Geometry check sheet. Reference: the model listing, model coordinates, mm. Face numbers are marked on the shaded views. A direction names the side the tool comes from. Give positions to 0.01 mm unless a question says otherwise; leave off trailing zeros. Loops run counter-clockwise (first coordinate to the right, second up) from the corner with the lowest first, then second, coordinate; pieces in that order, holes last.
1. Cross-section at C-C, the plane y = 33. Record the cut outline in (x, z), plus the area to 3 significant figures.
2. Cross-section at B-B, the plane z = -20.5. Record the cut outline in (x, y).
3. Cross-section at D-D, the plane x = -63. Record the cut outline in (y, z).
4. Go/stop test with flat-tipped pins: pin 1 Ø12 at (y, z) = (35, 22) entering from +X; pin 2 Ø15 at (x, z) = (90, -8.5) entering from +Y; pin 3 Ø6 at (y, z) = (46, -1) entering from +X; pin 4 Ø23 at (x, z) = (-95, 0) entering from -Y. Record where each tip stops, or that it passes through.
5. Release check for a two-part mould opening along X. For the marked faces 4 and 5 record: +X half, -X half, draft (parallel to the pull), parting line (faces both ways), or undercut.
6. Tool access check on the marked faces 1, 2 and 3. Record the directions out of +Z, -Z, +X, -X, +Y, -Y that give a thin tool (end or side, any length) a straight path to the whole face; none if there is none.
7. Cross-section at A-A, the plane x = 0. Record the cut outline in (y, z).
8. Material ranges on L1, parallel to X at y = 7.75, z = 0; L2, parallel to X at y = 16, z = -7; L3, parallel to Z at x = 95, y = 18, recorded low to high.
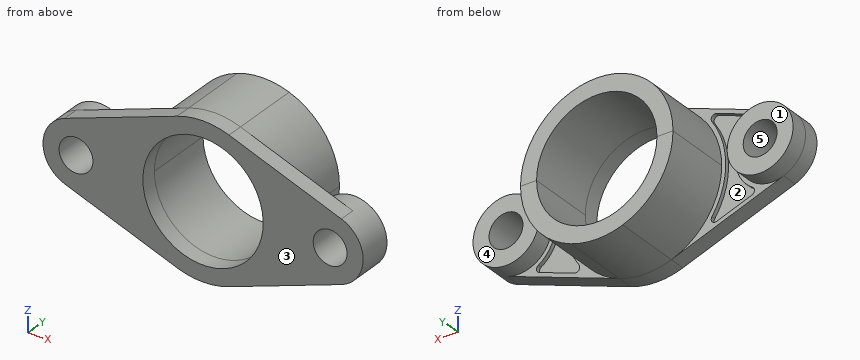
from build123d import *
from build123d.topology import SkipClean

# Parameters (mm, degrees)
SKETCH3_R                 = 12.666666667
SKETCH3_R_2               = 45
BOSS_EXTRUDE1_DEPTH       = 12
BOSS_EXTRUDE2_START       = 12
BOSS_EXTRUDE2_OUTLINE_R   = 24.666666667
BOSS_EXTRUDE2_OUTLINE_R_2 = 12.666666667
BOSS_EXTRUDE2_DEPTH       = 13
BOSS_EXTRUDE3_START       = 12
BOSS_EXTRUDE3_DEPTH       = 51
CUT_EXTRUDE1_DEPTH        = 3


# Read off the part's stored shape, not the designer's step: Boss-Extrude2
with BuildPart() as part:
    # Sketch3 → Boss-Extrude1 (new body)
    with BuildSketch(Plane(origin=(0, 0, 0), x_dir=(1, 0, 0), z_dir=(0, 1, 0))):
        with BuildLine():
            ThreePointArc((-103.395321637, 23.194029815), (-119.666666667, 0), (-103.395321637, -23.194029815))
            Line((-103.395321637, -23.194029815), (-19.4, -53.597014842))
            ThreePointArc((-19.4, -53.597014842), (0, -57), (19.4, -53.597014842))
            Line((19.4, -53.597014842), (103.395321637, -23.194029815))
            ThreePointArc((103.395321637, -23.194029815), (119.666666667, 0), (103.395321637, 23.194029815))
            Line((103.395321637, 23.194029815), (19.4, 53.597014842))
            ThreePointArc((19.4, 53.597014842), (0, 57), (-19.4, 53.597014842))
            Line((-19.4, 53.597014842), (-103.395321637, 23.194029815))
        make_face()
        with Locations(Location((-95, 0, 0), (0, 0, 270))):
            Circle(SKETCH3_R, mode=Mode.SUBTRACT)
        with Locations(Location((0, 0, 0), (0, 0, 270))):
            Circle(SKETCH3_R_2, mode=Mode.SUBTRACT)
        with Locations(Location((95, 0, 0), (0, 0, 270))):
            Circle(SKETCH3_R, mode=Mode.SUBTRACT)
    extrude(amount=BOSS_EXTRUDE1_DEPTH)

    # Boss-Extrude2 outline → Boss-Extrude2 (add)
    # profile 1 of 2: a face of its own
    with BuildSketch(Plane(origin=(0, 0, 0), x_dir=(1, 0, 0), z_dir=(0, 1, 0)).offset(BOSS_EXTRUDE2_START)):
        with Locations((-95, 0)):
            Circle(BOSS_EXTRUDE2_OUTLINE_R)
        with Locations((-95, 0)):
            Circle(BOSS_EXTRUDE2_OUTLINE_R_2, mode=Mode.SUBTRACT)
    # profile 2 of 2: a face of its own
    with BuildSketch(Plane(origin=(0, 0, 0), x_dir=(1, 0, 0), z_dir=(0, 1, 0)).offset(BOSS_EXTRUDE2_START)):
        with Locations((95, 0)):
            Circle(BOSS_EXTRUDE2_OUTLINE_R)
        with Locations((95, 0)):
            Circle(BOSS_EXTRUDE2_OUTLINE_R_2, mode=Mode.SUBTRACT)
    extrude(amount=BOSS_EXTRUDE2_DEPTH)

    # Sketch3<7> → Boss-Extrude3 (add)
    with SkipClean():  # the faces are left unmerged after this step: merging them gives an invalid solid
        with BuildSketch(Plane(origin=(0, 0, 0), x_dir=(1, 0, 0), z_dir=(0, 1, 0)).offset(BOSS_EXTRUDE3_START)):
            with BuildLine():
                ThreePointArc((-19.4, 53.597014842), (-46.662618872, 32.735302045), (-57, 0))
                Line((-57, 0), (-45, 0))
                ThreePointArc((-45, 0), (0, 45), (45, 0))
                Line((45, 0), (57, 0))
                ThreePointArc((57, 0), (46.662618872, 32.735302045), (19.4, 53.597014842))
                ThreePointArc((19.4, 53.597014842), (0, 57), (-19.4, 53.597014842))
            make_face()
            with BuildLine():
                Line((-45, 0), (-57, 0))
                ThreePointArc((-57, 0), (-46.662618872, -32.735302045), (-19.4, -53.597014842))
                ThreePointArc((-19.4, -53.597014842), (0, -57), (19.4, -53.597014842))
                ThreePointArc((19.4, -53.597014842), (46.662618872, -32.735302045), (57, 0))
                Line((57, 0), (45, 0))
                ThreePointArc((45, 0), (0, -45), (-45, 0))
            make_face()
        extrude(amount=BOSS_EXTRUDE3_DEPTH)

    # Sketch7 → Cut-Extrude1 (cut)
    with SkipClean():  # the faces are left unmerged after this step: merging them gives an invalid solid
        with BuildSketch(Plane(origin=(0, 12, 0), x_dir=(1, 0, 0), z_dir=(0, 1, 0))):
            with BuildLine():
                Line((79.495818927, -28.654228549), (53.157283033, -38.187737044))
                ThreePointArc((53.157283033, -38.187737044), (49.768127235, -37.208603561), (49.653552763, -33.682706216))
                ThreePointArc((49.653552763, -33.682706216), (60, 0), (49.653552763, 33.682706216))
                ThreePointArc((49.653552763, 33.682706216), (49.768127235, 37.208603561), (53.157283033, 38.187737044))
                Line((53.157283033, 38.187737044), (79.495818927, 28.654228549))
                ThreePointArc((79.495818927, 28.654228549), (81.456336863, 26.165352539), (80.091365245, 23.306159147))
                ThreePointArc((80.091365245, 23.306159147), (67.333333333, 0), (80.091365245, -23.306159147))
                ThreePointArc((80.091365245, -23.306159147), (81.456336863, -26.165352539), (79.495818927, -28.654228549))
            make_face()
            with BuildLine():
                Line((-53.157283033, 38.187737044), (-79.495818927, 28.654228549))
                ThreePointArc((-79.495818927, 28.654228549), (-81.456336863, 26.165352539), (-80.091365245, 23.306159147))
                ThreePointArc((-80.091365245, 23.306159147), (-67.333333333, 0), (-80.091365245, -23.306159147))
                ThreePointArc((-80.091365245, -23.306159147), (-81.456336863, -26.165352539), (-79.495818927, -28.654228549))
                Line((-79.495818927, -28.654228549), (-53.157283033, -38.187737044))
                ThreePointArc((-53.157283033, -38.187737044), (-49.768127235, -37.208603561), (-49.653552763, -33.682706216))
                ThreePointArc((-49.653552763, -33.682706216), (-60, 0), (-49.653552763, 33.682706216))
                ThreePointArc((-49.653552763, 33.682706216), (-49.768127235, 37.208603561), (-53.157283033, 38.187737044))
            make_face()
        extrude(amount=-CUT_EXTRUDE1_DEPTH, mode=Mode.SUBTRACT)


solid = part.part
Result:
1. outline: circle Ø114 at (0, 0); hole circle Ø90 at (0, 0)
1. area: 3,850 mm2
2. outline: (-108.72, 0) - (-40.06, 0) - (-40.06, 63) - (-53.19, 63) - (-53.19, 12) - (-56.39, 12) - (-56.39, 9) - (-76.42, 9) - (-76.42, 12) - (-81.28, 12) - (-81.28, 25) - (-108.72, 25) - close; (40.06, 0) - (108.72, 0) - (108.72, 25) - (81.28, 25) - (81.28, 12) - (76.42, 12) - (76.42, 9) - (56.39, 9) - (56.39, 12) - (53.19, 12) - (53.19, 63) - (40.06, 63) - close
3. outline: (0, -37.82) - (12, -37.82) - (12, -34.63) - (9, -34.63) - (9, 34.63) - (12, 34.63) - (12, 37.82) - (0, 37.82) - close
4. pin 1: stops at x = 54.71
4. pin 2: stops at y = 25
4. pin 3: stops at x = 57
4. pin 4: passes through
5. face 4: draft
5. face 5: undercut
6. face 1: +Z, -Z, -X, +Y
6. face 2: +Y
6. face 3: +Z, -Z, +X, -X, -Y
7. outline: (0, -57) - (63, -57) - (63, -45) - (0, -45) - close; (0, 45) - (63, 45) - (63, 57) - (0, 57) - close
8. L1: x = -119.67 to -107.67, -82.33 to -45, 45 to 82.33, 107.67 to 119.67
8. L2: x = -118.65 to -105.56, -84.44 to -71.35, -56.57 to -44.45, 44.45 to 56.57, 71.35 to 84.44, 105.56 to 118.65
8. L3: z = -24.67 to -12.67, 12.67 to 24.67
